Solid Edge part; units mm, degrees
sketch "Sketch1" plane through (-5.725, 0, 0) normal (1, 0, 0) x (0, 1, 0)
  arc A0 (-75.005, 301.708) -> (-89.005, 301.708) centre (-82.005, 301.708) cw
  line L0 (-89.005, 301.708) -> (-89.005, 383.708)
  line L1 (-89.005, 383.708) -> (-75.005, 397.708)
  line L2 (-75.005, 397.708) -> (-75.005, 301.708)
  line L3 (-79.305, 301.708) -> (-79.305, 358.708)
  arc A1 (-84.705, 301.708) -> (-79.305, 301.708) centre (-82.005, 301.708) ccw
  line L4 (-84.705, 358.708) -> (-84.705, 301.708)
  arc A2 (-79.305, 358.708) -> (-84.705, 358.708) centre (-82.005, 358.708) ccw
  dimension "D1" = 75.005
  dimension "D2" = 89.005
extrude "ExtrudedProtrusion_1" add sketch "Sketch1" along normal blind 2
extrude "Cutout1" [suppressed]
properties material "ABS Plastic, medium impact"
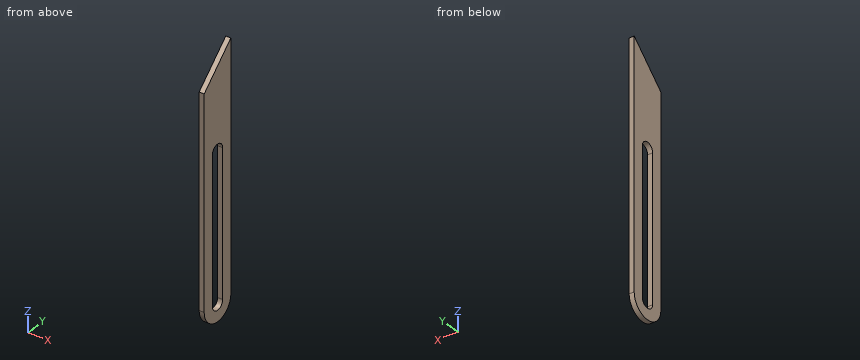
Model file for the job. Use its own axes, mm. Coordinates: 2 decimals unless noted, no trailing zeros. Order: outer loops, then holes, each group sorted by start corner. A loop starts at its lowest first (then second) coordinate and runs counter-clockwise, first axis right, second up. Notation, with made-up numbers: M 35.5,-8.5 L 70.5,-8.5 A19 ccw 70.5,18.5 Z; hole C -32.5,61 d3. An arc over 180 degrees is marked long. Return JSON: item names as keys, results as strings.
1. Drill centre lines: probe 1 along Y at (x, z) = (-4.85, 359) (3 decimals); probe 2 along Z at (x, y) = (-3.85, -80); probe 3 along Z at (x, y) = (-4.3, -87.5). Where is each one in solid material? Low to high.
Ans:
{"probe 1": "-89.005 to -84.689, -79.321 to -75.005", "probe 2": "295 to 299.9, 360.52 to 392.71", "probe 3": "297.37 to 385.21"}
2. Saw through at B-B (y = -80.25). Give the cut face in (x, z) (3 decimals), and give its area (3 significant figures).
Ans:
{"outline": "M -5.725,294.932 L -3.725,294.932 L -3.725,299.656 L -5.725,299.656 Z; M -5.725,360.76 L -3.725,360.76 L -3.725,392.463 L -5.725,392.463 Z", "area": "72.9 mm^2"}
3. Saw through at C-C (x = -4.7). Give the cut face in (y, z) (3 decimals).
Ans:
{"outline": "M -89.005,301.708 A7 ccw -75.005,301.708 L -75.005,397.708 L -89.005,383.708 Z; hole M -84.705,301.708 A2.7 ccw -79.305,301.708 L -79.305,358.708 A2.7 ccw -84.705,358.708 Z"}
4. Saw through at A-A (z = 357). Give the cut face in (x, y) (3 decimals), and give its area (3 significant figures).
Ans:
{"outline": "M -5.725,-89.005 L -3.725,-89.005 L -3.725,-84.705 L -5.725,-84.705 Z; M -5.725,-79.305 L -3.725,-79.305 L -3.725,-75.005 L -5.725,-75.005 Z", "area": "17.2 mm^2"}
5. Saw through at D-D (y = -86.5). Give the cut face in (x, z) (3 decimals).
Ans:
{"outline": "M -5.725,296.342 L -3.725,296.342 L -3.725,386.213 L -5.725,386.213 Z"}
